The listing builds one solid part. Answer for the finished solid, in the listing's coordinates (mm). Face numbers are marked on the shaded views. A direction names the side the tool comes from. Round coordinates to 2 decimals unless told otherwise and drop trailing zeros. Loops run counter-clockwise (first coordinate to the right, second up) from the corner with the lowest first, then second, coordinate; pieces in that order, holes last. Notation, with made-up numbers: (45, 52.5) -> (55, 52.5) arc R18 cw to (55, 66.5) -> close; hole circle Ø2 at (-36.5, 63). An arc over 180 degrees is marked (long way). Answer in a Markdown table with one row per item. Add a question column.
```python
from build123d import *

# Parameters (mm, degrees)
SKETCH1_W                = 60
SKETCH1_H                = 60
BOSS_EXTRUDE1_DEPTH      = 90
CUT_EXTRUDE4_DEPTH       = 100.498743711
CUT_EXTRUDE4_DEPTH_BACK  = 100.498743711
SKETCH5_R                = 2
SKETCH5_R_2              = 5
CUT_EXTRUDE6_DEPTH       = 113.249721603
CUT_EXTRUDE6_DEPTH_BACK  = 113.249721603
SKETCH7_W                = 62
SKETCH7_H                = 50
SKETCH8_R                = 19.3
CUT_EXTRUDE7_DEPTH       = 83
SKETCH10_W               = 5
SKETCH10_H               = 30.5
BOSS_EXTRUDE2_DEPTH      = 46
CHAMFER1_SIZE            = 48.010035871
CHAMFER1_SIZE_2          = 30
SKETCH11_W               = 14.5
SKETCH11_H               = 60
BOSS_EXTRUDE3_DEPTH      = 15
SKETCH12_W               = 14.5
SKETCH12_H               = 60
BOSS_EXTRUDE4_DEPTH      = 15
CHAMFER2_SIZE            = 15
CHAMFER2_SIZE2           = 52.65790913
BOSS_EXTRUDE5_DEPTH      = 15
BOSS_EXTRUDE5_DEPTH_BACK = 105
SKETCH13_W               = 14.5
SKETCH13_H               = 7.34209087
F_6_0MM_DOWEL_HOLE1_D    = 6


with BuildPart() as part:
    # Sketch1 → Boss-Extrude1 (new body)
    with BuildSketch(Plane.XY):
        Rectangle(SKETCH1_W, SKETCH1_H)
    extrude(amount=BOSS_EXTRUDE1_DEPTH)

    # Sketch5 → Cut-Extrude4 (cut, two sides: drawn at the far end of the back side and taken through both)
    with BuildSketch(Plane(origin=(0, 0, 0), x_dir=(-1, 0, 0), z_dir=(0, 0, -1)).offset(-CUT_EXTRUDE4_DEPTH_BACK)):
        with Locations((-8, 11)):
            Circle(SKETCH5_R)
        with Locations((8, 11)):
            Circle(SKETCH5_R)
        with Locations((8, -5)):
            Circle(SKETCH5_R)
        with Locations((-8, -5)):
            Circle(SKETCH5_R)
        with Locations((0, 3)):
            Circle(SKETCH5_R_2)
    extrude(amount=CUT_EXTRUDE4_DEPTH + CUT_EXTRUDE4_DEPTH_BACK, mode=Mode.SUBTRACT)

    # Sketch7 → Cut-Extrude6 (cut, two sides: drawn at the far end of the back side and taken through both)
    with BuildSketch(Plane.ZY.offset(30).offset(-CUT_EXTRUDE6_DEPTH_BACK)):
        with Locations((45, -9)):
            Rectangle(SKETCH7_W, SKETCH7_H)
    extrude(amount=CUT_EXTRUDE6_DEPTH + CUT_EXTRUDE6_DEPTH_BACK, mode=Mode.SUBTRACT)

    # Sketch8 → Cut-Extrude7 (cut)
    with BuildSketch(Plane(origin=(0, 0, 0), x_dir=(-1, 0, 0), z_dir=(0, 0, -1))):
        with Locations((0, 3)):
            Circle(SKETCH8_R)
    extrude(amount=-CUT_EXTRUDE7_DEPTH, mode=Mode.SUBTRACT)

    # Sketch10 → Boss-Extrude2 (add)
    with BuildSketch(Plane.XZ.offset(-16)):
        with Locations((-27.5, 60.75)):
            Rectangle(SKETCH10_W, SKETCH10_H)
        with Locations((-27.5, 29.25)):
            Rectangle(SKETCH10_W, SKETCH10_H)
        with Locations((27.5, 60.75)):
            Rectangle(SKETCH10_W, SKETCH10_H)
        with Locations((27.5, 29.25)):
            Rectangle(SKETCH10_W, SKETCH10_H)
    extrude(amount=BOSS_EXTRUDE2_DEPTH)

    # Chamfer1
    # the kernel refuses this chamfer: 48.010035871, 30 mm, written as the material it takes off along each edge
    with BuildSketch(Plane(origin=(99.122648056, -30, 44.5), x_dir=(0, 0.9997899140358645, 0.02049701910421798), z_dir=(-1, 0, 0))) as chamfer1_piece_1_section:
        Polygon((CHAMFER1_SIZE * 0.999789914041, CHAMFER1_SIZE * 0.0204970191043), (-CHAMFER1_SIZE_2 * 0.0204970191042, CHAMFER1_SIZE_2 * 0.999789914036), (0, 0), align=None)
    chamfer1_piece_1 = extrude(amount=253.245296112, mode=Mode.PRIVATE)
    chamfer1_piece_1 = split(chamfer1_piece_1, bisect_by=Plane(origin=(-27.5, 16, 34.735639976), z_dir=(0, -1, 0)), keep=Keep.TOP, mode=Mode.PRIVATE)
    add(chamfer1_piece_1, mode=Mode.SUBTRACT)
    with BuildSketch(Plane(origin=(-99.122648056, -30, 44.5), x_dir=(0, 0.9997899140358645, 0.02049701910421798), z_dir=(1, 0, 0))) as chamfer1_piece_2_section:
        Polygon((CHAMFER1_SIZE * 0.999789914041, -CHAMFER1_SIZE * 0.0204970191043), (-CHAMFER1_SIZE_2 * 0.0204970191042, -CHAMFER1_SIZE_2 * 0.999789914036), (0, 0), align=None)
    chamfer1_piece_2 = extrude(amount=253.245296112, mode=Mode.PRIVATE)
    chamfer1_piece_2 = split(chamfer1_piece_2, bisect_by=Plane(origin=(27.5, 16, 34.735639976), z_dir=(0, -1, 0)), keep=Keep.TOP, mode=Mode.PRIVATE)
    add(chamfer1_piece_2, mode=Mode.SUBTRACT)
    with BuildSketch(Plane(origin=(-99.122648056, -30, 45.5), x_dir=(0, 0.9997899140358645, -0.020497019104217966), z_dir=(1, 0, 0))) as chamfer1_piece_3_section:
        Polygon((CHAMFER1_SIZE * 0.999789914041, CHAMFER1_SIZE * 0.0204970191043), (-CHAMFER1_SIZE_2 * 0.0204970191042, CHAMFER1_SIZE_2 * 0.999789914036), (0, 0), align=None)
    chamfer1_piece_3 = extrude(amount=253.245296112, mode=Mode.PRIVATE)
    chamfer1_piece_3 = split(chamfer1_piece_3, bisect_by=Plane(origin=(27.5, 16, 55.264360024), z_dir=(0, -1, 0)), keep=Keep.TOP, mode=Mode.PRIVATE)
    add(chamfer1_piece_3, mode=Mode.SUBTRACT)
    with BuildSketch(Plane(origin=(99.122648056, -30, 45.5), x_dir=(0, -0.05243311939005598, 0.9986244379099823), z_dir=(-1, 0, 0))) as chamfer1_piece_4_section:
        Polygon((CHAMFER1_SIZE_2 * 0.99862443791, CHAMFER1_SIZE_2 * 0.0524331193901), (-CHAMFER1_SIZE * 0.0524331193903, CHAMFER1_SIZE * 0.998624437915), (0, 0), align=None)
    chamfer1_piece_4 = extrude(amount=253.245296112, mode=Mode.PRIVATE)
    chamfer1_piece_4 = split(chamfer1_piece_4, bisect_by=Plane(origin=(-27.5, 16, 55.264360024), z_dir=(0, -1, 0)), keep=Keep.TOP, mode=Mode.PRIVATE)
    add(chamfer1_piece_4, mode=Mode.SUBTRACT)

    # Sketch11 → Boss-Extrude3 (add)
    with BuildSketch(Plane.ZY.offset(30)):
        with Locations((7.25, 0)):
            Rectangle(SKETCH11_W, SKETCH11_H)
        with Locations((82.75, 0)):
            Rectangle(SKETCH11_W, SKETCH11_H)
    extrude(amount=BOSS_EXTRUDE3_DEPTH)

    # Sketch12 → Boss-Extrude4 (add)
    with BuildSketch(Plane(origin=(30, 0, 0), x_dir=(0, 0, -1), z_dir=(1, 0, 0))):
        with Locations((-82.75, 0)):
            Rectangle(SKETCH12_W, SKETCH12_H)
        with Locations((-7.25, 0)):
            Rectangle(SKETCH12_W, SKETCH12_H)
    extrude(amount=BOSS_EXTRUDE4_DEPTH)

    # Chamfer2
    chamfer2_edges = [part.edges().sort_by_distance(p)[0] for p in [
        (-45, 30, 7.25),
        (-45, 30, 82.75),
        (45, 30, 82.75),
        (45, 30, 7.25),
    ]]
    chamfer2_side = [part.faces().sort_by_distance(p)[0] for p in [
        (0, 30, 45),
    ]]
    chamfer(chamfer2_edges, length=CHAMFER2_SIZE, length2=CHAMFER2_SIZE2, reference=chamfer2_side[0])

    # Sketch13 → Boss-Extrude5 (add, two sides: drawn at the far end of the back side and taken through both)
    with BuildSketch(Plane(origin=(45, 0, 0), x_dir=(0, 0, -1), z_dir=(1, 0, 0)).offset(-BOSS_EXTRUDE5_DEPTH_BACK)):
        with Locations((-82.75, -26.328954565)):
            Rectangle(SKETCH13_W, SKETCH13_H)
        with Locations((-7.25, -26.328954565)):
            Rectangle(SKETCH13_W, SKETCH13_H)
    extrude(amount=BOSS_EXTRUDE5_DEPTH + BOSS_EXTRUDE5_DEPTH_BACK)

    # Ø6.0mm Dowel Hole1 (through all)
    with Locations(Plane(origin=(52.5, -22.65790913, 82.75), x_dir=(1, 0, 0), z_dir=(0, 1, 0))):
        with Locations((0, 0), (0, 75.5), (-105, 75.5), (-105, 0)):
            Hole(F_6_0MM_DOWEL_HOLE1_D / 2)


solid = part.part
```
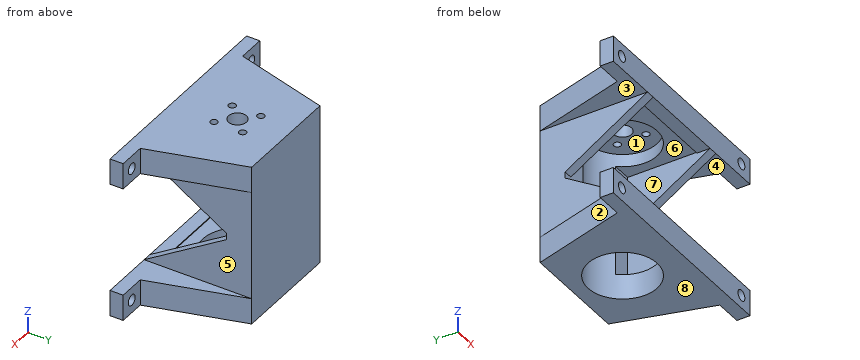
Item 1: Flat-ended cylindrical pins translate along their axes: P1, Ø16, axis at x = 55.5, z = 6.5, coming from the +Y side; P2, Ø23.5, axis at y = -10, z = 28.5, coming from the -X side; P3, Ø1.5, axis at x = 0, y = -10, coming from the -Z side; P4, Ø3.5, axis at x = 52.5, z = 7.25, coming from the +Y side. Find the tip coordinate at first contact, or state that the pin passes through.
Item 2: The mould has two halves that part along X. Classify the marked faces 5, 6, 7 and 8: +X half, -X half, draft (parallel to the pull), parting line (faces both ways), or undercut.
Item 3: Section C-C, the plane x = 3.5 is taken. Write down the section's boundary in (y, z), and give its area (3 significant figures).
Item 4: Section A-A, the plane x = 52.5 is taken. Write down the section's boundary in (y, z).
Item 5: Section D-D, the plane y = 3 is taken. Give the number of separate pieces and of enclosed holes in the cut face, and give its area (3 significant figures).
Item 6: Section B-B, the plane z = 52 is taken. Write down the section's boundary in (x, y) (3 decimals).
Item 7: For the marked faces 1, 2, 3 and 4, determine the directions among +Z, -Z, +X, -X, +Y, -Y from which every point of the face is accessible in a straight line to the end or side of a thin tool.
Item 8: Consider L1, parallel to Z at x = 52.5, y = -27; L2, parallel to X at y = -28.5, z = 82.75; L3, parallel to X at y = -8.5, z = 72. Determine where each line is inside the solid, lowest interval first. Write a range as from..to.
Here are the results:
| question | item | result |
|---|---|---|
| 1 | P1 | stops at y = -22.66 |
| 1 | P2 | stops at x = -30 |
| 1 | P3 | stops at z = 83 |
| 1 | P4 | passes through |
| 2 | face 5 | +X half |
| 2 | face 6 | undercut |
| 2 | face 7 | undercut |
| 2 | face 8 | draft |
| 3 | outline | (-30, 0) -> (-15.98, 0) -> (-15.98, 14) -> (-22.66, 14) -> (-22.66, 14.5) -> (-30, 14.5) -> close; (-30, 75.5) -> (-22.66, 75.5) -> (-22.66, 76) -> (-15.98, 76) -> (-15.98, 83) -> (-0.57, 83) -> (-0.57, 90) -> (-30, 90) -> close; (6.57, 83) -> (21.98, 83) -> (21.98, 0) -> (30, 0) -> (30, 90) -> (6.57, 90) -> close |
| 3 | area | 1,340 mm² |
| 4 | outline | (-30, 0) -> (-22.66, 0) -> (-22.66, 4.25) -> (-30, 4.25) -> close; (-30, 10.25) -> (-22.66, 10.25) -> (-22.66, 14.5) -> (-30, 14.5) -> close; (-30, 75.5) -> (-22.66, 75.5) -> (-22.66, 79.75) -> (-30, 79.75) -> close; (-30, 85.75) -> (-22.66, 85.75) -> (-22.66, 90) -> (-30, 90) -> close |
| 5 | separate pieces | 4 |
| 5 | enclosed holes | 0 |
| 5 | area | 1,670 mm² |
| 6 | outline | (-30, 7.608) -> (-25, 7.608) -> (-25, 16) -> (-14.265, 16) arc R19.3 cw to (14.265, 16) -> (25, 16) -> (25, 7.608) -> (30, 7.608) -> (30, 30) -> (-30, 30) -> close |
| 7 | face 1 | -Z |
| 7 | face 2 | +Z, -Z, -X, +Y |
| 7 | face 3 | -X, +Y, -Y |
| 7 | face 4 | +X, +Y, -Y |
| 8 | L1 | z = 0..4.25, 10.25..14.5, 75.5..79.75, 85.75..90 |
| 8 | L2 | x = -60..-55.5, -49.5..49.5, 55.5..60 |
| 8 | L3 | x = -30..-25, 25..30 |
